Autodesk Inventor part; units mm, degrees
ref_plane "YZ Plane" through (0, 0, 0) normal (1, 0, 0) x (0, 1, 0)
ref_plane "XZ Plane" through (0, 0, 0) normal (0, 1, 0) x (-1, 0, 0)
ref_plane "XY Plane" through (0, 0, 0) normal (0, 0, 1) x (1, 0, 0)
sketch "Sketch1" plane through (0, 0, 0) normal (0, 1, 0) x (-1, 0, 0)
  circle A0 centre (0, 0) radius 5
  line L0 (2.2293, 3.2) -> (-2.2293, 3.2)
  line L1 (-3.2, 2.2293) -> (-3.2, -2.2293)
  line L2 (-2.2293, -3.2) -> (2.2293, -3.2)
  line L3 (3.2, -2.2293) -> (3.2, 2.2293)
  arc A1 (3.2, 2.2293) -> (2.2293, 3.2) centre (0, 0) ccw
  arc A2 (2.2293, -3.2) -> (3.2, -2.2293) centre (0, 0) ccw
  arc A3 (-2.2293, 3.2) -> (-3.2, 2.2293) centre (0, 0) ccw
  arc A4 (-3.2, -2.2293) -> (-2.2293, -3.2) centre (0, 0) ccw
  dimension "d0" = 10
  dimension "d2" = 3.2
  dimension "d3" = 3.2
  dimension "d5" = 6.4
extrude "Extrusion1" add sketch "Sketch1" along normal blind 1.5875
fillet "Fillet1" radius 0.3 18 edges at (0, 1.5875, 3.2) (0, 0, 3.2) (-2.7577, 0, 2.7577) (-2.7577, 1.5875, 2.7577) (-3.2, 1.5875, 0) (-3.2, 0, 0) (-2.7577, 0, -2.7577) (0, 0, -3.2) (0, 1.5875, -3.2) (-2.7577, 1.5875, -2.7577) (2.7577, 1.5875, -2.7577) (3.2, 1.5875, 0) (2.7577, 1.5875, 2.7577) (2.7577, 0, -2.7577) (3.2, 0, 0) (2.7577, 0, 2.7577) (5, 0, 0) (5, 1.5875, 0)
fillet "Fillet1" radius 0.1 8 edges at (2.2293, 0.7937, 3.2) (3.2, 0.7937, 2.2293) (3.2, 0.7937, -2.2293) (-3.2, 0.7937, -2.2293) (-2.2293, 0.7937, -3.2) (-3.2, 0.7937, 2.2293) (-2.2293, 0.7937, 3.2) (2.2293, 0.7937, -3.2)
properties part number "Spacer High Strength" material "Acetal Resin, Black"
Check sheet for the modelled part. Datum: model origin and axes. Units: mm. A direction names the side the tool comes from. Round coordinates to 2 decimals unless told otherwise and drop trailing zeros. Order: outer loops, then holes, each group sorted by start corner. A loop starts at its lowest first (then second) coordinate and runs counter-clockwise, first axis right, second up. Notation, with made-up numbers: (18.25, -10) - (36.25, -10) arc R25 ccw to (36.25, 9) - close; hole circle Ø2 at (2.25, 11). An arc over 180 degrees is marked (long way). Answer as CSV lines item,"result". Start each with the question number.
1) Scan lines: probe 1 along Z at (x, y) = (0, 0.7); probe 2 along X at (y, z) = (1.45, 0.5); probe 3 along X at (y, z) = (1.4, 0.25). Record each from-to range of solid material in increasing order.
2) Draft check along X on faces 3 (the face through (-3.2, 1, 0)), 4 (the face through (1.08, 0.79, 4.88)), 5 (the face through (0, 1.588, 4)). Enter one of: +X half, -X half, draft (parallel to the pull), parting line (faces both ways), or undercut.
3) Section check C-C (y = 0.7). Record the cut outline in (x, z).
4) Section check B-B (z = 0). Record the cut outline in (x, y).
5) Section check A-A (x = 0). Record the cut outline in (y, z).
6) Tool access check on faces 1 (the face through (0, 0, 4)), 2 (the face through (0, 1, -3.2)). Record the directions out of +Z, -Z, +X, -X, +Y, -Y that give a thin tool (end or side, any length) a straight path to the whole face; none if there is none.
Determined:
1,probe 1,"-5 to -3.2, 3.2 to 5"
1,probe 2,"-4.93 to -3.25, 3.25 to 4.93"
1,probe 3,"-4.97 to -3.22, 3.22 to 4.97"
2,face 3,"undercut"
2,face 4,"parting line"
2,face 5,"draft"
3,outline,"circle Ø10 at (0, 0); hole (-3.2, -2.2) arc R0.1 ccw to (-3.18, -2.26) arc R3.9 ccw to (-2.26, -3.18) arc R0.1 ccw to (-2.2, -3.2) - (2.2, -3.2) arc R0.1 ccw to (2.26, -3.18) arc R3.9 ccw to (3.18, -2.26) arc R0.1 ccw to (3.2, -2.2) - (3.2, 2.2) arc R0.1 ccw to (3.18, 2.26) arc R3.9 ccw to (2.26, 3.18) arc R0.1 ccw to (2.2, 3.2) - (-2.2, 3.2) arc R0.1 ccw to (-2.26, 3.18) arc R3.9 ccw to (-3.18, 2.26) arc R0.1 ccw to (-3.2, 2.2) - close"
4,outline,"(-5, 0.3) arc R0.3 ccw to (-4.7, 0) - (-3.5, 0) arc R0.3 ccw to (-3.2, 0.3) - (-3.2, 1.29) arc R0.3 ccw to (-3.5, 1.59) - (-4.7, 1.59) arc R0.3 ccw to (-5, 1.29) - close; (3.2, 0.3) arc R0.3 ccw to (3.5, 0) - (4.7, 0) arc R0.3 ccw to (5, 0.3) - (5, 1.29) arc R0.3 ccw to (4.7, 1.59) - (3.5, 1.59) arc R0.3 ccw to (3.2, 1.29) - close"
5,outline,"(0, -4.7) arc R0.3 ccw to (0.3, -5) - (1.29, -5) arc R0.3 ccw to (1.59, -4.7) - (1.59, -3.5) arc R0.3 ccw to (1.29, -3.2) - (0.3, -3.2) arc R0.3 ccw to (0, -3.5) - close; (0, 3.5) arc R0.3 ccw to (0.3, 3.2) - (1.29, 3.2) arc R0.3 ccw to (1.59, 3.5) - (1.59, 4.7) arc R0.3 ccw to (1.29, 5) - (0.3, 5) arc R0.3 ccw to (0, 4.7) - close"
6,face 1,"+Z, -Z, +X, -X, -Y"
6,face 2,"+Y, -Y"
